Model file for the job. Use its own axes, mm. A direction names the side the tool comes from. Give positions to 0.01 mm unless a question says otherwise; leave off trailing zeros. Loops run counter-clockwise (first coordinate to the right, second up) from the corner with the lowest first, then second, coordinate; pieces in that order, holes last. Notation, with made-up numbers: (22.25, 15) -> (81.25, 15) arc R23 cw to (81.25, 34) -> close; hole circle Ø5 at (-27.75, -18). An arc over 180 degrees is marked (long way). Use CSV: the item, a comma, the result in double quotes. Start each with the question number.
(1) Cut at B-B on y = 20. State how many separate pieces and enclosed holes the cut face has, then the cut area to 3 significant figures.
(2) Cut at A-A on x = 15.5. Write the cut outline in (y, z).
(3) Flat gauge pins, fed straight in: pin 1 (1.5 mm diameter, centred on x = 34.5, y = 24.5, fed in from -Z); pin 2 (5.5 mm diameter, centred on x = 32.5, y = 20, fed in from +Z); pin 3 (5 mm diameter, centred on x = 32, y = 20.5, fed in from -Z); pin 4 (10 mm diameter, centred on x = 35.5, y = 26, fed in from -Z). Where does each tip first touch, or does it go through?
(4) Pull direction Y, two halves, no side cores. Call faces 1 (the flat face through (11.365, 13.812, -2.028)), 2 (the cylindrical face through (2.199, 21.053, -15.604)), 3 (the cylindrical face through (28.88, 2.46, -23.51)): pulls with the +Y half, pulls with the -Y half, needs draft (parallel to the pull), parting line crosses it, or undercut.
(5) Cut at C-C on x = 5.8. Write the cut outline in (y, z) (3 decimals).
(6) Drill centre lines: probe 1 along X at (y, z) = (2.05, -23); probe 2 along Z at (x, y) = (30.5, 1.15); probe 3 along X at (y, z) = (14, -1.25) (3 decimals). Where is each one in solid material? Low to high.
(7) 3-axis set-ups, long thin cutter, end or side, ignore diameter. For faces 4 (the cylindrical face through (33.096, 23.727, -8.288)), 5 (the flat face through (40.754, 20.776, -16.168)), 6 (the flat face through (5, 29, -6)): which of +Z, -Z, +X, -X, +Y, -Y reach the whole face in a straight line?
from build123d import *
from build123d.topology import SkipClean

# Parameters (mm, degrees)
SKETCH1_W                           = 42
SKETCH1_H                           = 28
BOSS_EXTRUDE1_DEPTH                 = 5
SKETCH2_W                           = 42
SKETCH2_H                           = 4
BOSS_EXTRUDE2_DEPTH                 = 32
TAP_DRILL_FOR_M1_6X0_35_TAP1_D      = 1.25
M3_CLEARANCE_HOLE1_D                = 3.4
BOSS_EXTRUDE3_DEPTH                 = 2.5
BOSS_EXTRUDE4_DEPTH                 = 2.5
FILLET2_R                           = 1
SKETCH9_R                           = 3.25
CUT_EXTRUDE1_DEPTH                  = 1
SKETCH10_R                          = 2.44
CUT_EXTRUDE2_DEPTH                  = 62.302528496
SKETCH11_R                          = 0.625
BOSS_EXTRUDE5_DEPTH                 = 6.2
CUT_EXTRUDE3_DEPTH                  = 61.901559914
BOSS_EXTRUDE6_REACH                 = 64.586
BOSS_EXTRUDE8_START                 = 7
SKETCH16_R                          = 4.75
SKETCH16_R_2                        = 3.25
BOSS_EXTRUDE8_DEPTH                 = 7
SKETCH17_R                          = 1.5
CUT_EXTRUDE4_DEPTH                  = 0.5
TAP_DRILL_FOR_M1_6X0_35_TAP2_REACH  = 58.001
TAP_DRILL_FOR_M1_6X0_35_TAP2_BORE_R = 0.625
SKETCH21_W                          = 2
SKETCH21_H                          = 8
CUT_EXTRUDE5_DEPTH                  = 6.2


with BuildPart() as part:
    # Sketch1 → Boss-Extrude1 (new body)
    with BuildSketch(Plane(origin=(0, 0, 0), x_dir=(1, 0, 0), z_dir=(0, 1, 0))):
        with Locations((21, 14)):
            Rectangle(SKETCH1_W, SKETCH1_H)
    extrude(amount=BOSS_EXTRUDE1_DEPTH)

    # Sketch2 → Boss-Extrude2 (add)
    with BuildSketch(Plane(origin=(0, 5, 0), x_dir=(1, 0, 0), z_dir=(0, 1, 0))):
        with Locations((21, 2)):
            Rectangle(SKETCH2_W, SKETCH2_H)
    extrude(amount=BOSS_EXTRUDE2_DEPTH)

    # Tap Drill for M1.6x0.35 Tap1 (through all)
    with Locations(Plane(origin=(0, 0, -4), x_dir=(-1, 0, 0), z_dir=(0, 0, -1))):
        with Locations((-22, 14.5), (-5.8, 14.5)):
            Hole(TAP_DRILL_FOR_M1_6X0_35_TAP1_D / 2)

    # M3 Clearance Hole1 (through all)
    with Locations(Plane(origin=(0, 5, 0), x_dir=(1, 0, 0), z_dir=(0, 1, 0))):
        with Locations((15.5, 23), (30.5, 23), (30.5, 10), (15.5, 10)):
            Hole(M3_CLEARANCE_HOLE1_D / 2)

    # Sketch7 → Boss-Extrude3 (add)
    with BuildSketch(Plane.ZY):
        Polygon((-28, 5), (-4, 37), (-4, 5), align=None)
    extrude(amount=-BOSS_EXTRUDE3_DEPTH)

    # Sketch8 → Boss-Extrude4 (add)
    with BuildSketch(Plane(origin=(42, 0, 0), x_dir=(0, 0, -1), z_dir=(1, 0, 0))):
        Polygon((28, 5), (4, 37), (4, 5), align=None)
    extrude(amount=-BOSS_EXTRUDE4_DEPTH)

    # Fillet2
    fillet2_edges = [part.edges().sort_by_distance(p)[0] for p in [
        (0, 37, -2),
        (42, 37, -2),
        (2.5, 21, -16),
        (0, 21, -16),
        (39.5, 21, -16),
        (42, 21, -16),
        (0, 2.5, -28),
        (42, 2.5, -28),
    ]]
    fillet(fillet2_edges, radius=FILLET2_R)

    # Sketch9 → Cut-Extrude1 (cut)
    with BuildSketch(Plane(origin=(0, 0, -4), x_dir=(-1, 0, 0), z_dir=(0, 0, -1))):
        with Locations((-32.5, 20)):
            Circle(SKETCH9_R)
    extrude(amount=-CUT_EXTRUDE1_DEPTH, mode=Mode.SUBTRACT)

    # Sketch10 → Cut-Extrude2 (cut, through all)
    with BuildSketch(Plane(origin=(0, 0, -3), x_dir=(-1, 0, 0), z_dir=(0, 0, -1))):
        with Locations((-32.5, 20)):
            Circle(SKETCH10_R)
    extrude(amount=-CUT_EXTRUDE2_DEPTH, mode=Mode.SUBTRACT)

    # Sketch11 → Boss-Extrude5 (add)
    # profile 1 of 2: a face of its own
    with SkipClean():  # the faces are left unmerged after this step: merging them gives an invalid solid
        with BuildSketch(Plane(origin=(0, 0, -4), x_dir=(-1, 0, 0), z_dir=(0, 0, -1))):
            with BuildLine():
                Line((-3.65, 37), (-4.65, 37))
                Line((-4.65, 37), (-4.65, 14.989897949))
                ThreePointArc((-4.65, 14.989897949), (-7.05, 14.5), (-4.65, 14.010102051))
                Line((-4.65, 14.010102051), (-3.65, 14.010102051))
                Line((-3.65, 14.010102051), (-3.65, 37))
            make_face()
            with Locations((-5.8, 14.5)):
                Circle(SKETCH11_R, mode=Mode.SUBTRACT)
        # profile 2 of 2: a face of its own
        with BuildSketch(Plane(origin=(0, 0, -4), x_dir=(-1, 0, 0), z_dir=(0, 0, -1))):
            with BuildLine():
                Line((-24.15, 37), (-23.15, 37))
                Line((-23.15, 37), (-23.15, 14.989897949))
                ThreePointArc((-23.15, 14.989897949), (-20.75, 14.5), (-23.15, 14.010102051))
                Line((-23.15, 14.010102051), (-24.15, 14.010102051))
                Line((-24.15, 14.010102051), (-24.15, 37))
            make_face()
            with Locations((-22, 14.5)):
                Circle(SKETCH11_R, mode=Mode.SUBTRACT)
        extrude(amount=BOSS_EXTRUDE5_DEPTH)
    add(part.part.scale(1), mode=Mode.REPLACE)  # the faces are merged on a copy

    # Sketch13 → Cut-Extrude3 (cut, through all)
    with BuildSketch(Plane(origin=(0, 0, -4), x_dir=(-1, 0, 0), z_dir=(0, 0, -1))):
        Polygon((-13.9, 28.708767963), (-8.9, 22.75), (-8.9, 16.75), (-13.9, 10.791232037), (-18.9, 16.75), (-18.9, 22.75), align=None)
    extrude(amount=-CUT_EXTRUDE3_DEPTH, mode=Mode.SUBTRACT)

    # Sketch14 → Boss-Extrude6 (add, up to next)
    with BuildSketch(Plane(origin=(0, 37, 0), x_dir=(1, 0, 0), z_dir=(0, 1, 0)), mode=Mode.PRIVATE) as boss_extrude6_sk1:
        Polygon((23.15, 10.2), (21.15, 4), (23.15, 4), align=None)
    boss_extrude6_tool1 = extrude(boss_extrude6_sk1.sketch, amount=-BOSS_EXTRUDE6_REACH, mode=Mode.PRIVATE) - part.part
    # Sketch14 → Boss-Extrude6 (add, up to next)
    with BuildSketch(Plane(origin=(0, 37, 0), x_dir=(1, 0, 0), z_dir=(0, 1, 0)), mode=Mode.PRIVATE) as boss_extrude6_sk2:
        Polygon((4.65, 10.2), (6.65, 4), (4.65, 4), align=None)
    boss_extrude6_tool2 = extrude(boss_extrude6_sk2.sketch, amount=-BOSS_EXTRUDE6_REACH, mode=Mode.PRIVATE) - part.part
    add(boss_extrude6_tool1.solids().sort_by_distance((22.483333, 37, -6.066667))[0])
    add(boss_extrude6_tool2.solids().sort_by_distance((5.316667, 37, -6.066667))[0])

    # Sketch16 → Boss-Extrude8 (add)
    with SkipClean():  # the faces are left unmerged after this step: merging them gives an invalid solid
        with BuildSketch(Plane(origin=(0, 0, -4), x_dir=(-1, 0, 0), z_dir=(0, 0, -1)).offset(BOSS_EXTRUDE8_START)):
            with Locations(Location((-32.5, 20, 0), (0, 0, 180))):
                Circle(SKETCH16_R)
            with Locations((-32.5, 20)):
                Circle(SKETCH16_R_2, mode=Mode.SUBTRACT)
        extrude(amount=-BOSS_EXTRUDE8_DEPTH)

    # Sketch17 → Cut-Extrude4 (cut)
    with SkipClean():  # the faces are left unmerged after this step: merging them gives an invalid solid
        with BuildSketch(Plane(origin=(0, 24.75, 0), x_dir=(1, 0, 0), z_dir=(0, 1, 0))):
            with Locations(Location((32.5, 8.1, 0), (0, 0, 270))):
                Circle(SKETCH17_R)
        extrude(amount=-CUT_EXTRUDE4_DEPTH, mode=Mode.SUBTRACT)

    # Tap Drill for M1.6x0.35 Tap2 bore → Tap Drill for M1.6x0.35 Tap2 (cut, up to next)
    with BuildSketch(Plane(origin=(0, 24.25, 0), x_dir=(1, 0, 0), z_dir=(0, 1, 0)), mode=Mode.PRIVATE) as tap_drill_for_m1_6x0_35_tap2_sk1:
        with Locations((32.5, 8.1)):
            Circle(TAP_DRILL_FOR_M1_6X0_35_TAP2_BORE_R)
    tap_drill_for_m1_6x0_35_tap2_tool1 = extrude(tap_drill_for_m1_6x0_35_tap2_sk1.sketch, amount=-TAP_DRILL_FOR_M1_6X0_35_TAP2_REACH, mode=Mode.PRIVATE) & part.part
    add(tap_drill_for_m1_6x0_35_tap2_tool1.solids().sort_by_distance((32.5, 24.25, -8.1))[0], mode=Mode.SUBTRACT)

    # Sketch21 → Cut-Extrude5 (cut)
    with BuildSketch(Plane(origin=(0, 0, -10.2), x_dir=(-1, 0, 0), z_dir=(0, 0, -1))):
        with Locations((-5.65, 33)):
            Rectangle(SKETCH21_W, SKETCH21_H)
        with Locations((-22.15, 33)):
            Rectangle(SKETCH21_W, SKETCH21_H)
    extrude(amount=-CUT_EXTRUDE5_DEPTH, mode=Mode.SUBTRACT)


solid = part.part
Check result:
1,separate pieces,"3"
1,enclosed holes,"0"
1,area,"215 mm²"
2,outline,"(0, -28) -> (5, -28) -> (5, -24.7) -> (0, -24.7) -> close; (0, -21.3) -> (5, -21.3) -> (5, -11.7) -> (0, -11.7) -> close; (0, -8.3) -> (5, -8.3) -> (5, -4) -> (12.7, -4) -> (12.7, 0) -> (0, 0) -> close; (26.8, -4) -> (37, -4) -> (37, 0) -> (26.8, 0) -> close"
3,pin 1,"z = -11"
3,pin 2,"z = 0"
3,pin 3,"z = -3"
3,pin 4,"z = -13.81"
4,face 1,"undercut"
4,face 2,"pulls with the +Y half"
4,face 3,"needs draft"
5,outline,"(0, -28) -> (5, -28) -> (5, -4) -> (13.25, -4) -> (13.25, -10.2) -> (13.875, -10.2) -> (13.875, 0) -> (0, 0) -> close; (15.125, -10.2) -> (15.75, -10.2) -> (15.75, -6.635) -> (29, -6.635) -> (29, -4) -> (37, -4) -> (37, 0) -> (15.125, 0) -> close"
6,probe 1,"0 to 13.8, 17.2 to 28.8, 32.2 to 42"
6,probe 2,"-28 to -24.7, -21.3 to -11.7, -8.3 to 0"
6,probe 3,"0 to 5.425, 6.175 to 11.208, 16.592 to 21.625, 22.375 to 42"
7,face 4,"+Y"
7,face 5,"-Z, +X, +Y"
7,face 6,"-Z, +Y"
